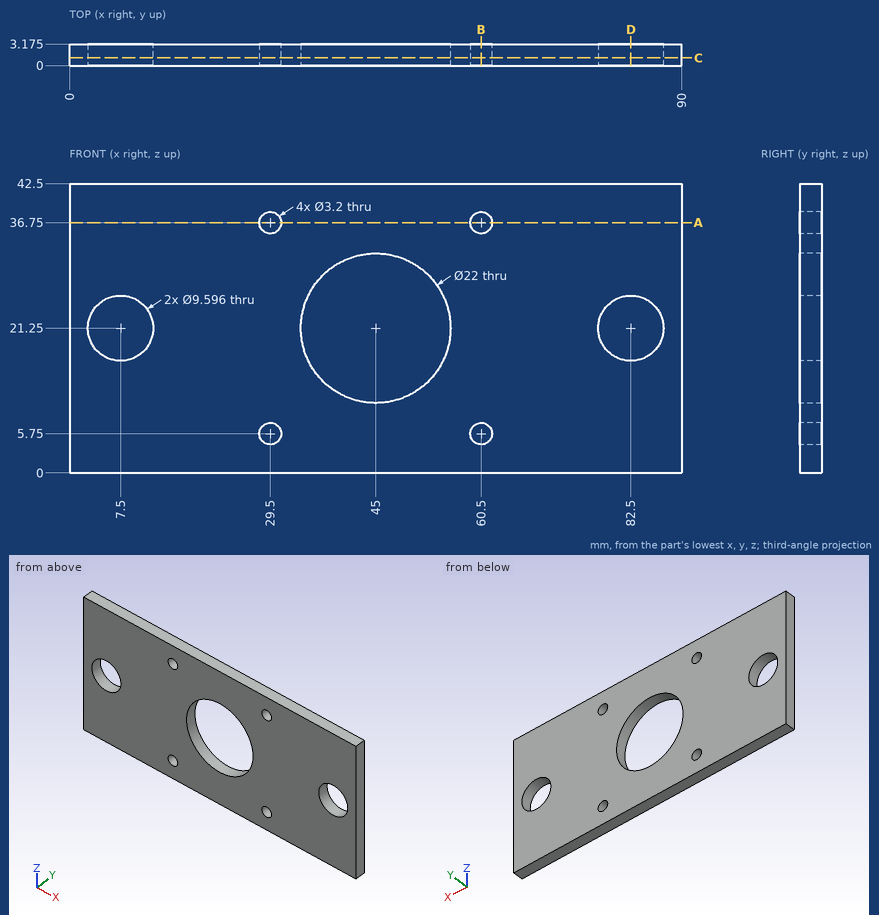
The figure shows three views and two pictorial views of one solid part (mm, origin at its lowest corner). Answer the questions. Give positions to 0.01 mm unless a question says otherwise; leave off trailing zeros. Order: outer loops, then holes, each group sorted by start corner. A loop starts at its lowest first (then second) coordinate and runs counter-clockwise, first axis right, second up. Notation, with made-up numbers: M 69,72 L 83,72 A12 cw 83,80 Z; hole C 13,61 d6. An arc over 180 degrees is marked long. Return JSON: item names as keys, results as strings.
1) Section C-C, the plane y = 1.15 is taken. Write down the section's boundary in (x, z).
Resolved:
{"outline": "M 0,0 L 90,0 L 90,42.5 L 0,42.5 Z; hole C 7.5,21.25 d9.6; hole C 29.5,5.75 d3.2; hole C 29.5,36.75 d3.2; hole C 45,21.25 d22; hole C 60.5,5.75 d3.2; hole C 60.5,36.75 d3.2; hole C 82.5,21.25 d9.6"}
2) Section B-B, the plane x = 60.5 is taken. Write down the section's boundary in (y, z) (3 decimals).
Resolved:
{"outline": "M 0,0 L 3.175,0 L 3.175,4.15 L 0,4.15 Z; M 0,7.35 L 3.175,7.35 L 3.175,35.15 L 0,35.15 Z; M 0,38.35 L 3.175,38.35 L 3.175,42.5 L 0,42.5 Z"}
3) Straight lines are drawn through the part: line 1 along Z through (x, y) = (29.5, 0.7); line 2 along X through (y, z) = (1.4, 21.25); line 3 along Z through (x, y) = (82.5, 1.8). For each, find the intervals that lie inside material, in ascending order. Write a range as [from, to].
Resolved:
{"line 1": "[0, 4.15], [7.35, 35.15], [38.35, 42.5]", "line 2": "[0, 2.7], [12.3, 34], [56, 77.7], [87.3, 90]", "line 3": "[0, 16.45], [26.05, 42.5]"}
4) Section D-D, the plane x = 82.5 is taken. Write down the section's boundary in (y, z) (3 decimals), plus the area to 3 significant figures.
Resolved:
{"outline": "M 0,0 L 3.175,0 L 3.175,16.452 L 0,16.452 Z; M 0,26.048 L 3.175,26.048 L 3.175,42.5 L 0,42.5 Z", "area": "104 mm^2"}
5) Section A-A, the plane z = 36.75 is taken. Write down the section's boundary in (x, y) (3 decimals), plus the area to 3 significant figures.
Resolved:
{"outline": "M 0,0 L 27.9,0 L 27.9,3.175 L 0,3.175 Z; M 31.1,0 L 58.9,0 L 58.9,3.175 L 31.1,3.175 Z; M 62.1,0 L 90,0 L 90,3.175 L 62.1,3.175 Z", "area": "265 mm^2"}
6) This flat-tipped pin is pushed along its axis until it touches: pin 1 (2.5 mm diameter, centred on x = 60.5, z = 5.75, fed in from +Y). Where does it stop, or does it pass through?
Resolved:
{"pin 1": "through"}
